from build123d import *

# Parameters (mm, degrees)
F0_W     = 76.2
F0_H     = 152.4
F1_DEPTH = 15.24
F2_W     = 68.948708
F2_H     = 143.428072
F3_DEPTH = 5.08
F4_R     = 2.54


with BuildPart() as f1:
    # F0 (on Front) → F1 (new body)
    with BuildSketch(Plane.XZ):
        Rectangle(F0_W, F0_H)
    extrude(amount=F1_DEPTH)

    # F2 (on face) → F3 (cut)
    with BuildSketch(Plane(origin=(0, 0, 0), x_dir=(-1, 0, 0), z_dir=(0, 1, 0))):
        Rectangle(F2_W, F2_H)
    extrude(amount=-F3_DEPTH, mode=Mode.SUBTRACT)

    # F4
    f4_edges = [f1.edges().sort_by_distance(p)[0] for p in [
        (-38.1, -7.62, -76.2),
        (38.1, -7.62, -76.2),
        (38.1, -7.62, 76.2),
        (-38.1, -7.62, 76.2),
        (-38.1, -15.24, 0),
        (38.1, -15.24, 0),
        (0, -15.24, 76.2),
        (0, -15.24, -76.2),
    ]]
    fillet(f4_edges, radius=F4_R)


solid = f1.part
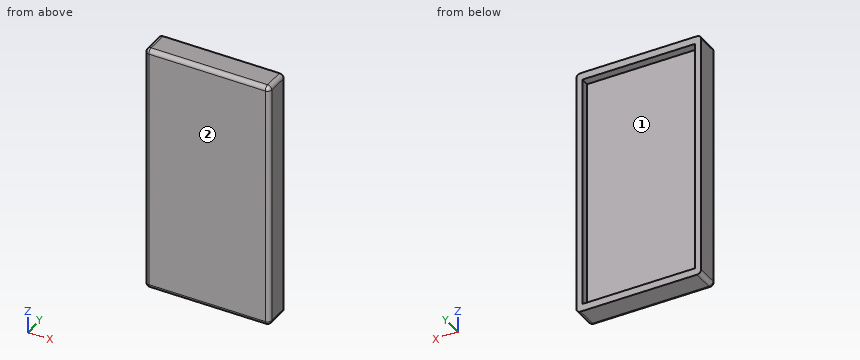
Verification items for the finished model (mm, model axes). Face numbers are marked on the shaded views. Coordinates: 2 decimals unless noted, no trailing zeros. Order: outer loops, then holes, each group sorted by start corner. A loop starts at its lowest first (then second) coordinate and runs counter-clockwise, first axis right, second up. Notation, with made-up numbers: (87.25, 29) -> (95.25, 29) arc R12 cw to (95.25, 38) -> close; hole circle Ø8 at (23.25, 19.25). An arc over 180 degrees is marked (long way). Put each result on its own line as item: value. Start each with the question number.
1. Mould release check, pull along X, two halves, no side actions. Record for the marked faces 1 and 2: released by +X, released by -X, zero draft, split by the parting line, or undercut.
2. Go/stop test with a flat-tipped pin: pin 1 Ø3 at (x, z) = (-21.5, -25.5) entering from +Y. Record where the tip stops, or that it passes through.
3. Cross-section at B-B, the plane y = -2.5. Record the boundary of the cut face in (x, z), then the cut area to 3 significant figures.
4. Material ranges on L1, parallel to Z at x = -18, y = -4.5; L2, parallel to X at y = -3.5, z = 21; L3, parallel to Y at x = 20, z = -70, recorded low to high. Write a range as [from, to].
5. Cross-section at C-C, the plane x = 9.5. Record the boundary of the cut face in (y, z).
6. Cross-section at A-A, the plane z = -6. Record the boundary of the cut face in (x, y).
Computed:
1. face 1: undercut
1. face 2: zero draft
2. pin 1: y = -5.08
3. outline: (-38.1, -73.66) arc R2.54 ccw to (-35.56, -76.2) -> (35.56, -76.2) arc R2.54 ccw to (38.1, -73.66) -> (38.1, 73.66) arc R2.54 ccw to (35.56, 76.2) -> (-35.56, 76.2) arc R2.54 ccw to (-38.1, 73.66) -> close; hole (-34.47, -71.71) -> (34.47, -71.71) -> (34.47, 71.71) -> (-34.47, 71.71) -> close
3. area: 1,720 mm2
4. L1: [-76.2, -71.71], [71.71, 76.2]
4. L2: [-38.1, -34.47], [34.47, 38.1]
4. L3: [-15.24, -5.08]
5. outline: (-15.24, -73.66) arc R2.54 ccw to (-12.7, -76.2) -> (0, -76.2) -> (0, -71.71) -> (-5.08, -71.71) -> (-5.08, 71.71) -> (0, 71.71) -> (0, 76.2) -> (-12.7, 76.2) arc R2.54 ccw to (-15.24, 73.66) -> close
6. outline: (-38.1, -12.7) arc R2.54 ccw to (-35.56, -15.24) -> (35.56, -15.24) arc R2.54 ccw to (38.1, -12.7) -> (38.1, 0) -> (34.47, 0) -> (34.47, -5.08) -> (-34.47, -5.08) -> (-34.47, 0) -> (-38.1, 0) -> close
